Autodesk Inventor part; units mm, degrees
ref_plane "Work Plane1" through (0, 0, 0) normal (0, 0, 1) x (1, 0, 0)
ref_plane "YZ Plane" through (0, 0, 0) normal (1, 0, 0) x (0, 1, 0)
ref_plane "XZ Plane" through (0, 0, 0) normal (0, 1, 0) x (-1, 0, 0)
ref_plane "Work Plane1" through (0, 0, 0) normal (0, 0, 1) x (1, 0, 0)
ref_plane "Work Plane2" through (-15.674, 29.0262, 3.81) normal (0, 0, 1) x (1, 0, 0)
sketch "Sketch2" plane through (-15.674, 29.0262, 3.81) normal (0, 0, 1) x (1, 0, 0)
  circle A0 centre (0, 0) radius 5.08
  circle A1 centre (0, 0) radius 2.286
  circle A2 centre (44.7003, -13.3522) radius 5.08
  circle A3 centre (44.7003, -13.3522) radius 2.286
  circle A4 centre (31.3481, -58.0524) radius 2.286
  circle A5 centre (31.3481, -58.0524) radius 5.08
  circle A6 centre (-13.3522, -44.7003) radius 2.286
  circle A7 centre (-13.3522, -44.7003) radius 5.08
  circle A8 centre (15.674, -29.0262) radius 38.0678
  circle A9 centre (15.674, -29.0262) radius 3.937
  dimension "d7" = 7.874
extrude "Extrusion2" add sketch "Sketch2" along normal blind 2.54 contours A0 | A7 | A5 | A2 | A8
properties part number "cover"
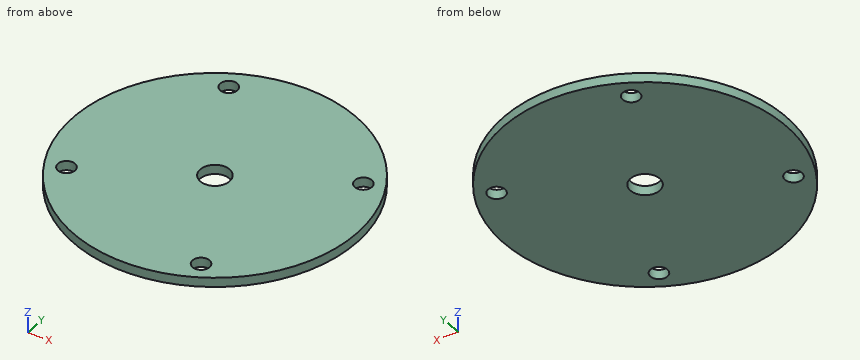
Input: part model. Units: mm. Frame: model coordinates. Coordinates: 2 decimals unless noted, no trailing zeros. Write each loop counter-clockwise with the first axis right and the second up, starting at its lowest first coordinate (ties: lowest second). Pieces come first, ordered by that corner, then holes. Notation, with made-up numbers: (83, 36) - (89, 36) arc R16 cw to (89, 50) - close; hole circle Ø11 at (53.5, 76.25). An arc over 180 degrees is marked (long way). Put each result on its own line as item: value. Start each with the question number.
1) Cut plane D-D (x = 21). Return the cut outline in (y, z).
2) Ray query, L1, parallel to X at y = 15, z = 6.1; L2, parallel to Y at x = 14, z = 4.2. Return the intervals inside material, ascending.
3) Cut plane C-C (z = 4.6). Return the cut outline in (x, y), plus the area to 3 significant figures.
4) Cut plane A-A (y = 0). Return the cut outline in (x, z), plus the area to 3 significant figures.
5) Contact query for a flat-ended pin moving along its axis: pin 1 (1.5 mm diameter, centred on y = -3.5, z = 4, fed in from +X). Output: stop coordinate, or through.
Resolved:
1. outline: (-31.75, 3.81) - (31.75, 3.81) - (31.75, 6.35) - (-31.75, 6.35) - close
2. L1: x = -34.99 to 26.84, 31.21 to 34.99
2. L2: y = -35.4 to -30.58, -27.47 to 35.4
3. outline: circle Ø76.14 at (0, 0); hole circle Ø4.57 at (-29.03, -15.67); hole circle Ø4.57 at (-15.67, 29.03); hole circle Ø7.87 at (0, 0); hole circle Ø4.57 at (15.67, -29.03); hole circle Ø4.57 at (29.03, 15.67)
3. area: 4,440 mm2
4. outline: (-38.07, 3.81) - (-3.94, 3.81) - (-3.94, 6.35) - (-38.07, 6.35) - close; (3.94, 3.81) - (38.07, 3.81) - (38.07, 6.35) - (3.94, 6.35) - close
4. area: 173 mm2
5. pin 1: stops at x = 37.97
